from build123d import *

# Parameters (mm, degrees)
SKETCH1_W           = 80
SKETCH1_H           = 40
BOSS_EXTRUDE1_DEPTH = 3
SKETCH2_R           = 6
CUT_EXTRUDE1_DEPTH  = 65.101482042
SKETCH5_W           = 4
SKETCH5_H           = 20
SKETCH5_W_2         = 51.247459446
CUT_EXTRUDE2_DEPTH  = 65.101482042
FILLET1_R           = 5
SKETCH6_W           = 3
SKETCH6_H           = 5
BOSS_EXTRUDE2_DEPTH = 3
LPATTERN1_COUNT     = 3
LPATTERN1_PITCH     = 30


with BuildPart() as part:
    # Sketch1 → Boss-Extrude1 (new body)
    with BuildSketch(Plane(origin=(0, 0, 0), x_dir=(0, 0, -1), z_dir=(1, 0, 0))):
        with Locations((10, 20)):
            Rectangle(SKETCH1_W, SKETCH1_H)
    extrude(amount=BOSS_EXTRUDE1_DEPTH)

    # Sketch2 → Cut-Extrude1 (cut, through all)
    with BuildSketch(Plane(origin=(3, 0, 0), x_dir=(0, 0, -1), z_dir=(1, 0, 0))):
        with Locations((-10, 20)):
            Circle(SKETCH2_R)
    extrude(amount=-CUT_EXTRUDE1_DEPTH, mode=Mode.SUBTRACT)

    # Sketch5 → Cut-Extrude2 (cut, through all)
    with BuildSketch(Plane.ZY):
        with BuildLine():
            Line((-28, 30), (-28, 40))
            Line((-28, 40), (-38, 40))
            Line((-38, 40), (-38, 30))
            ThreePointArc((-38, 30), (-33, 25), (-28, 30))
        make_face()
        with Locations((-48, 30)):
            Rectangle(SKETCH5_W, SKETCH5_H)
        with Locations((5.623729723, 30)):
            Rectangle(SKETCH5_W_2, SKETCH5_H)
    extrude(amount=-CUT_EXTRUDE2_DEPTH, mode=Mode.SUBTRACT)

    # Fillet1
    # the kernel refuses this fillet: 5 mm, written as the material it adds along each edge
    with BuildSketch(Plane(origin=(0, 20, -20), x_dir=(0, 1, 0), z_dir=(1, 0, 0))) as fillet1_piece_1:
        with BuildLine():
            CenterArc((FILLET1_R, FILLET1_R), FILLET1_R, 180, 90)
            Line((0, FILLET1_R), (0, 0))
            Line((0, 0), (FILLET1_R, 0))
        make_face()
    extrude(amount=3)
    # the kernel refuses this fillet: 5 mm, written as the material it takes off along each edge
    with BuildSketch(Plane(origin=(-12.5, 40, -46), x_dir=(0, -1, 0), z_dir=(1, 0, 0)), Plane(origin=(-12.5, 40, -20), x_dir=(0, 0, -1), z_dir=(1, 0, 0)), Plane(origin=(15.5, 20, 30), x_dir=(0, -1, 0), z_dir=(-1, 0, 0))) as fillet1_2_piece_1:
        with BuildLine():
            CenterArc((FILLET1_R, -FILLET1_R), FILLET1_R, 90, 90)
            Line((0, -FILLET1_R), (0, 0))
            Line((0, 0), (FILLET1_R, 0))
        make_face()
    extrude(amount=28, mode=Mode.SUBTRACT)
    with BuildSketch(Plane(origin=(-12.247448714, 20, -50), x_dir=(0, -1, 0), z_dir=(1, 0, 0))) as fillet1_2_piece_2:
        with BuildLine():
            CenterArc((4.898979486, -5), FILLET1_R, 90, 78.463040967)
            Line((0, -4), (0, 0))
            Line((0, 0), (4.898979486, 0))
        make_face()
    extrude(amount=27.494897428, mode=Mode.SUBTRACT)

    # Sketch6 → Boss-Extrude2 (add)
    with BuildSketch(Plane.XZ):
        with Locations((1.5, 20)):
            Rectangle(SKETCH6_W, SKETCH6_H)
    boss_extrude2 = extrude(amount=BOSS_EXTRUDE2_DEPTH)

    # LPattern1: Boss-Extrude2 ×3
    with Locations(*[(0, 0, -i * LPATTERN1_PITCH) for i in range(1, LPATTERN1_COUNT)]):
        add(boss_extrude2)


solid = part.part
The listing builds one solid part. Answer for the finished solid, in the listing's coordinates (mm). A direction names the side the tool comes from. Give positions to 0.01 mm unless a question says otherwise; leave off trailing zeros. Order: outer loops, then holes, each group sorted by start corner. A loop starts at its lowest first (then second) coordinate and runs counter-clockwise, first axis right, second up. Notation, with made-up numbers: (60, 13.5) - (92, 13.5) arc R21 ccw to (92, 20.5) - close; hole circle Ø9 at (73, 6.5). An arc over 180 degrees is marked (long way). One line per item, written item: value. Start each with the question number.
1) A cutting plane is placed at D-D on y = 37. Give the vertices of the cut face in (x, z), then the cut area to 3 significant figures.
2) Find the intervals of material crossed by L1, parallel to Z at x = 0.1, y = 32; L2, parallel to Z at x = 0.75, y = 15; L3, parallel to Y at x = 2.75, z = -10, in increasing order.
3) A cutting plane is placed at C-C on z = 10. Give the vertices of the cut face in (x, y).
4) A tool of negligible diameter and unlimited length cuts with its end or side. For faces 4 (the face through (1, 0, -46)), 5 (the face through (1, 27, -46)), 6 (the face through (1, 0, 5)), 7 (the face through (1, 0, 26)), from which of +Z, -Z, +X, -X, +Y, -Y can it reach the whole face along a straight path? Write none if from no direction.
5) Given pin 1 Ø1.5 at (x, z) = (2, 10) entering from -Y; pin 2 Ø1.5 at (x, z) = (2, 22.5) entering from +Y; pin 3 Ø0.9 at (x, y) = (1, 36) entering from +Z, each flat-ended and moving along its own axis, determine where each tip first touches the part or whether it passes through.
6) The mould has two halves that part along Z. Classify faces 1 (the face through (1, -3, -40)), 2 (the face through (1, 25, -33)), 3 (the face through (1, 38, -45)): released by +Z, released by -Z, zero draft, split by the parting line, or undercut.
7) A cutting plane is placed at B-B on y = 32.5. Give the vertices of the cut face in (x, z).
Answer sheet:
1. outline: (0, -45.58) - (3, -45.58) - (3, -38) - (0, -38) - close; (0, -28) - (3, -28) - (3, -20.42) - (0, -20.42) - close
1. area: 45.5 mm2
2. L1: z = -46 to -38, -28 to -20
2. L2: z = -50 to 6.68, 13.32 to 30
2. L3: y = -3 to 20
3. outline: (0, 0) - (3, 0) - (3, 14) - (0, 14) - close
4. face 4: -Z, +X, -X, -Y
4. face 5: -Z, +X, -X, +Y
4. face 6: +X, -X, -Y
4. face 7: +Z, +X, -X, -Y
5. pin 1: stops at y = 0
5. pin 2: stops at y = 20
5. pin 3: stops at z = -20.03
6. face 1: zero draft
6. face 2: undercut
6. face 3: released by -Z
7. outline: (0, -46) - (3, -46) - (3, -38) - (0, -38) - close; (0, -28) - (3, -28) - (3, -20) - (0, -20) - close
